The drawing under review shows one solid part. Ordinate dimensions are in mm from its lowest x, y, z. A direction names the side the tool comes from. Round coordinates to 2 decimals unless told otherwise and drop trailing zeros. Order: outer loops, then holes, each group sorted by start corner. A loop starts at its lowest first (then second) coordinate and runs counter-clockwise, first axis right, second up. Notation, with made-up numbers: M 88.5,4.5 L 144.5,4.5 A26 ccw 144.5,43.5 Z; hole C 78.5,-3.75 d8. An arc over 180 degrees is marked long. Answer as a JSON object with one key per item and string values. Group by question number.
1. Mouldability with a two-part tool opening along Z and no side actions: class the marked faces 1, 2 and 3 as released by +Z, released by -Z, zero draft, split by the parting line, or undercut.
2. Add section C-C on z = 8.5. State the section outline as (x, y) points, and give its area (3 significant figures).
3. To check wall thickness, follow probe 1 along Y at (x, z) = (20, 43.15); probe 2 along Z at (x, y) = (32, 49); probe 3 along Y at (x, z) = (26, 11). State the ranges of each line that lie inside material, in increasing order. Write a range as [from, to].
4. Machinability: for the marked faces 4 and 5, which of the approach directions +Z, -Z, +X, -X, +Y, -Y give a long, thin tool a straight path to every point of the face, cutting with its end or side? Answer none if there is none.
5. Add section A-A on y = 15. State the section outline as (x, z) points.
6. Add section B-B on x = 29. State the section outline as (y, z) points.
7. Add section D-D on y = 51.5. State the section outline as (x, z) points.
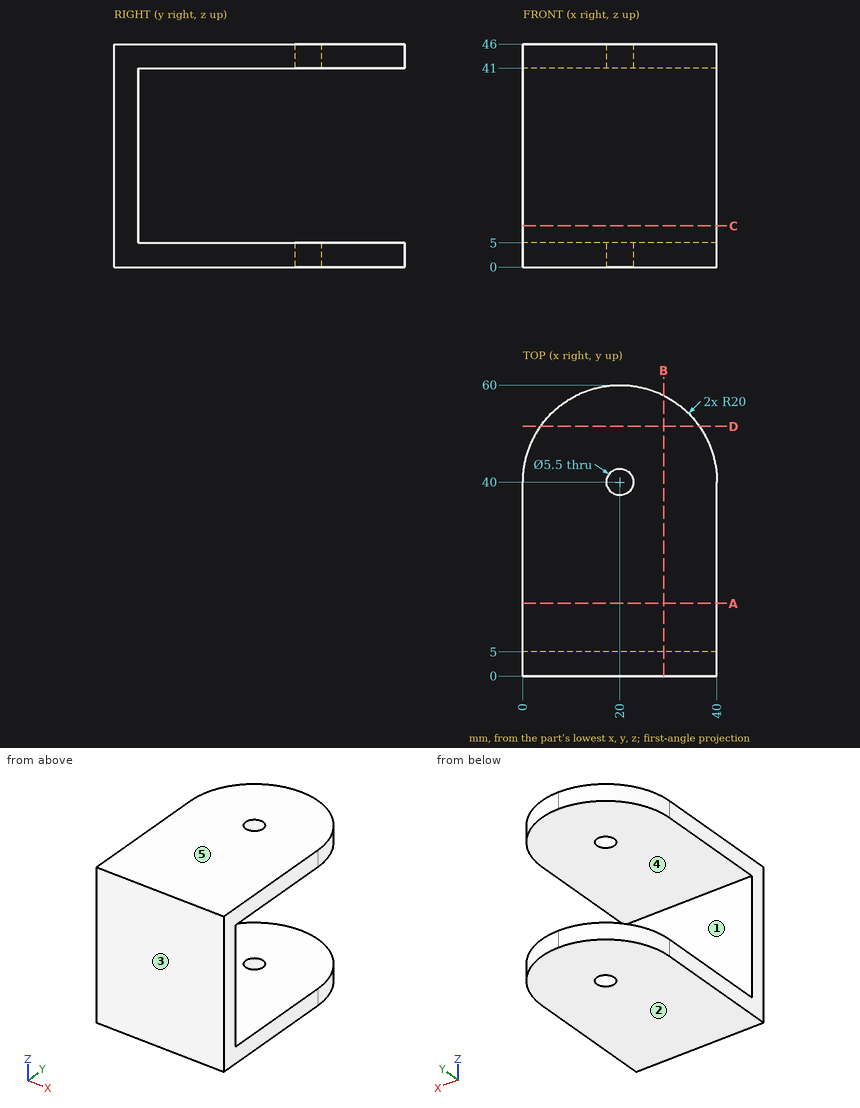
Recorded:
{
 "1": {"face 1": "undercut", "face 2": "released by -Z", "face 3": "zero draft"},
 "2": {"outline": "M 0,0 L 40,0 L 40,5 L 0,5 Z", "area": "200 mm²"},
 "3": {"probe 1": "y = [0, 37.25], [42.75, 60]", "probe 2": "z = [0, 5], [41, 46]", "probe 3": "y = [0, 5]"},
 "4": {"face 4": "+X, -X, +Y", "face 5": "+Z, +X, -X, +Y, -Y"},
 "5": {"outline": "M 0,0 L 40,0 L 40,5 L 0,5 Z; M 0,41 L 40,41 L 40,46 L 0,46 Z"},
 "6": {"outline": "M 0,0 L 57.86,0 L 57.86,5 L 5,5 L 5,41 L 57.86,41 L 57.86,46 L 0,46 Z"},
 "7": {"outline": "M 3.64,0 L 36.36,0 L 36.36,5 L 3.64,5 Z; M 3.64,41 L 36.36,41 L 36.36,46 L 3.64,46 Z"}
}
